from build123d import *

# Parameters (mm, degrees)
SKETCH1_W                      = 552
SKETCH1_H                      = 450
BOSS_EXTRUDE1_DEPTH            = 100
SKETCH2_W                      = 97
SKETCH2_H                      = 450
CUT_EXTRUDE1_DEPTH             = 90
SKETCH3_W                      = 450
SKETCH3_H                      = 97
CUT_EXTRUDE2_DEPTH             = 90
BOSS_EXTRUDE2_DEPTH            = 3
SKETCH5_W                      = 360
SKETCH5_H                      = 100
CUT_EXTRUDE3_DEPTH             = 542.403325206
SKETCH6_W                      = 20
SKETCH6_H                      = 3
BOSS_EXTRUDE3_DEPTH            = 90
SKETCH7_W                      = 20
SKETCH7_H                      = 3
BOSS_EXTRUDE4_DEPTH            = 90
CUT_EXTRUDE4_REACH             = 653.826
SKETCH9_W                      = 75
SKETCH9_H                      = 133
CUT_EXTRUDE5_DEPTH             = 538.285771261
CUT_EXTRUDE6_REACH             = 655.929
CUT_EXTRUDE7_REACH             = 653.826
CUT_EXTRUDE8_REACH             = 655.929
SKETCH13_W                     = 56
SKETCH13_H                     = 10
CUT_EXTRUDE9_DEPTH             = 1
SKETCH14_W                     = 56
SKETCH14_H                     = 10
CUT_EXTRUDE10_DEPTH            = 1
SKETCH15_W                     = 56
SKETCH15_H                     = 10
CUT_EXTRUDE11_DEPTH            = 1
SKETCH16_W                     = 56
SKETCH16_H                     = 10
CUT_EXTRUDE12_DEPTH            = 1
F_3_3_3_3_DIAMETER_HOLE1_D     = 3.3
F_3_3_3_3_DIAMETER_HOLE1_DEPTH = 2
F_17_0_17_DIAMETER_HOLE1_D     = 17
F_17_0_17_DIAMETER_HOLE1_DEPTH = 3
F_17_0_17_DIAMETER_HOLE2_D     = 17
F_17_0_17_DIAMETER_HOLE2_DEPTH = 103
FILLET1_R                      = 3


with BuildPart() as part:
    # Sketch1 → Boss-Extrude1 (new body)
    with BuildSketch(Plane(origin=(0, 120.173044165, 0), x_dir=(1, 0, 0), z_dir=(0, 1, 0))):
        with Locations((0, -225)):
            Rectangle(SKETCH1_W, SKETCH1_H)
    extrude(amount=-BOSS_EXTRUDE1_DEPTH)

    # Sketch2 → Cut-Extrude1 (cut)
    with BuildSketch(Plane(origin=(-273, 0, 0), x_dir=(0, -1, 0), z_dir=(-1, 0, 0))):
        with Locations((-68.673044165, 225)):
            Rectangle(SKETCH2_W, SKETCH2_H)
    extrude(amount=-CUT_EXTRUDE1_DEPTH, mode=Mode.SUBTRACT)

    # Sketch3 → Cut-Extrude2 (cut)
    with BuildSketch(Plane(origin=(273, 0, 0), x_dir=(0, 0, -1), z_dir=(1, 0, 0))):
        with Locations((-225, 68.673044165)):
            Rectangle(SKETCH3_W, SKETCH3_H)
    extrude(amount=-CUT_EXTRUDE2_DEPTH, mode=Mode.SUBTRACT)

    # Sketch4 → Boss-Extrude2 (add)
    with BuildSketch(Plane.XZ.offset(-20.173044165)):
        Polygon((-273, 360), (-273, 0), (-276, 0), (-276, 450), (-273, 450), (-273, 380), (-183, 380), (-183, 450), (183, 450), (183, 90), (273, 90), (273, 450), (276, 450), (276, 0), (273, 0), (273, 70), (183, 70), (183, 0), (-183, 0), (-183, 360), align=None)
    extrude(amount=BOSS_EXTRUDE2_DEPTH)

    # Sketch5 → Cut-Extrude3 (cut, through all)
    with BuildSketch(Plane(origin=(0, 0, 0), x_dir=(-1, 0, 0), z_dir=(0, 0, -1))):
        with Locations((0, 70.173044165)):
            Rectangle(SKETCH5_W, SKETCH5_H)
    extrude(amount=-CUT_EXTRUDE3_DEPTH, mode=Mode.SUBTRACT)

    # Sketch6 → Boss-Extrude3 (add)
    with BuildSketch(Plane(origin=(-273, 0, 0), x_dir=(0, 0, -1), z_dir=(1, 0, 0))):
        with Locations((-80, 18.673044165)):
            Rectangle(SKETCH6_W, SKETCH6_H)
    extrude(amount=BOSS_EXTRUDE3_DEPTH)

    # Sketch7 → Boss-Extrude4 (add)
    with BuildSketch(Plane.ZY.offset(-273)):
        with Locations((370, 18.673044165)):
            Rectangle(SKETCH7_W, SKETCH7_H)
    extrude(amount=BOSS_EXTRUDE4_DEPTH)

    # Sketch8 → Cut-Extrude4 (cut, up to next)
    with BuildSketch(Plane(origin=(-180, 0, 0), x_dir=(0, 0, -1), z_dir=(1, 0, 0)), mode=Mode.PRIVATE) as cut_extrude4_sk1:
        with BuildLine():
            Line((-440, 48.173044165), (-420, 48.173044165))
            ThreePointArc((-420, 48.173044165), (-413, 55.173044165), (-420, 62.173044165))
            Line((-420, 62.173044165), (-440, 62.173044165))
            ThreePointArc((-440, 62.173044165), (-447, 55.173044165), (-440, 48.173044165))
        make_face()
    cut_extrude4_tool1 = extrude(cut_extrude4_sk1.sketch, amount=-CUT_EXTRUDE4_REACH, mode=Mode.PRIVATE) & part.part
    add(cut_extrude4_tool1.solids().sort_by_distance((-180, 55.173044, 430))[0], mode=Mode.SUBTRACT)

    # Sketch9 → Cut-Extrude5 (cut, through all)
    with BuildSketch(Plane.XZ.offset(-117.173044165)):
        with Locations((-225, 225)):
            Rectangle(SKETCH9_W, SKETCH9_H)
    extrude(amount=-CUT_EXTRUDE5_DEPTH, mode=Mode.SUBTRACT)

    # Sketch10 → Cut-Extrude6 (cut, up to next)
    with BuildSketch(Plane.ZY.offset(183), mode=Mode.PRIVATE) as cut_extrude6_sk1:
        with BuildLine():
            Line((10, 48.173044165), (30, 48.173044165))
            ThreePointArc((30, 48.173044165), (37, 55.173044165), (30, 62.173044165))
            Line((30, 62.173044165), (10, 62.173044165))
            ThreePointArc((10, 62.173044165), (3, 55.173044165), (10, 48.173044165))
        make_face()
    cut_extrude6_tool1 = extrude(cut_extrude6_sk1.sketch, amount=-CUT_EXTRUDE6_REACH, mode=Mode.PRIVATE) & part.part
    add(cut_extrude6_tool1.solids().sort_by_distance((-183, 55.173044, 20))[0], mode=Mode.SUBTRACT)

    # Sketch11 → Cut-Extrude7 (cut, up to next)
    with BuildSketch(Plane.ZY.offset(-180), mode=Mode.PRIVATE) as cut_extrude7_sk1:
        with BuildLine():
            Line((440, 62.173044165), (420, 62.173044165))
            ThreePointArc((420, 62.173044165), (413, 55.173044165), (420, 48.173044165))
            Line((420, 48.173044165), (440, 48.173044165))
            ThreePointArc((440, 48.173044165), (447, 55.173044165), (440, 62.173044165))
        make_face()
    cut_extrude7_tool1 = extrude(cut_extrude7_sk1.sketch, amount=-CUT_EXTRUDE7_REACH, mode=Mode.PRIVATE) & part.part
    add(cut_extrude7_tool1.solids().sort_by_distance((180, 55.173044, 430))[0], mode=Mode.SUBTRACT)

    # Sketch12 → Cut-Extrude8 (cut, up to next)
    with BuildSketch(Plane(origin=(183, 0, 0), x_dir=(0, 0, -1), z_dir=(1, 0, 0)), mode=Mode.PRIVATE) as cut_extrude8_sk1:
        with BuildLine():
            Line((-10, 62.173044165), (-30, 62.173044165))
            ThreePointArc((-30, 62.173044165), (-37, 55.173044165), (-30, 48.173044165))
            Line((-30, 48.173044165), (-10, 48.173044165))
            ThreePointArc((-10, 48.173044165), (-3, 55.173044165), (-10, 62.173044165))
        make_face()
    cut_extrude8_tool1 = extrude(cut_extrude8_sk1.sketch, amount=-CUT_EXTRUDE8_REACH, mode=Mode.PRIVATE) & part.part
    add(cut_extrude8_tool1.solids().sort_by_distance((183, 55.173044, 20))[0], mode=Mode.SUBTRACT)

    # Sketch13 → Cut-Extrude9 (cut)
    with BuildSketch(Plane(origin=(0, 20.173044165, 0), x_dir=(-1, 0, 0), z_dir=(0, 1, 0))):
        with Locations((233, 80)):
            Rectangle(SKETCH13_W, SKETCH13_H)
    extrude(amount=-CUT_EXTRUDE9_DEPTH, mode=Mode.SUBTRACT)

    # Sketch14 → Cut-Extrude10 (cut)
    with BuildSketch(Plane(origin=(0, 20.173044165, 0), x_dir=(-1, 0, 0), z_dir=(0, 1, 0))):
        with Locations((233, 370)):
            Rectangle(SKETCH14_W, SKETCH14_H)
    extrude(amount=-CUT_EXTRUDE10_DEPTH, mode=Mode.SUBTRACT)

    # Sketch15 → Cut-Extrude11 (cut)
    with BuildSketch(Plane(origin=(0, 20.173044165, 0), x_dir=(-1, 0, 0), z_dir=(0, 1, 0))):
        with Locations((-233, 370)):
            Rectangle(SKETCH15_W, SKETCH15_H)
    extrude(amount=-CUT_EXTRUDE11_DEPTH, mode=Mode.SUBTRACT)

    # Sketch16 → Cut-Extrude12 (cut)
    with BuildSketch(Plane(origin=(0, 20.173044165, 0), x_dir=(-1, 0, 0), z_dir=(0, 1, 0))):
        with Locations((-233, 80)):
            Rectangle(SKETCH16_W, SKETCH16_H)
    extrude(amount=-CUT_EXTRUDE12_DEPTH, mode=Mode.SUBTRACT)

    # Ø3.3 (3.3) Diameter Hole1
    with Locations(Plane(origin=(0, 19.173044165, 0), x_dir=(1, 0, 0), z_dir=(0, 1, 0))):
        with Locations((-254.5, -80), (-211.5, -80), (-254.5, -370), (-211.5, -370), (211.5, -370), (254.5, -370), (211.5, -80), (254.5, -80)):
            Hole(F_3_3_3_3_DIAMETER_HOLE1_D / 2, depth=F_3_3_3_3_DIAMETER_HOLE1_DEPTH)

    # Ø17.0 (17) Diameter Hole1
    with Locations(Plane(origin=(0, 120.173044165, 0), x_dir=(1, 0, 0), z_dir=(0, 1, 0))):
        with Locations((225, -95)):
            Hole(F_17_0_17_DIAMETER_HOLE1_D / 2, depth=F_17_0_17_DIAMETER_HOLE1_DEPTH)

    # Ø17.0 (17) Diameter Hole2
    with Locations(Plane(origin=(0, 120.173044165, 0), x_dir=(1, 0, 0), z_dir=(0, 1, 0))):
        with Locations((-225, -100), (-225, -125), (-225, -325), (-225, -350)):
            Hole(F_17_0_17_DIAMETER_HOLE2_D / 2, depth=F_17_0_17_DIAMETER_HOLE2_DEPTH)

    # Fillet1
    fillet1_edges = [part.edges().sort_by_distance(p)[0] for p in [
        (-180, 120.173044165, 225),
        (180, 120.173044165, 225),
        (276, 120.173044165, 225),
        (-276, 120.173044165, 225),
    ]]
    fillet(fillet1_edges, radius=FILLET1_R)


solid = part.part
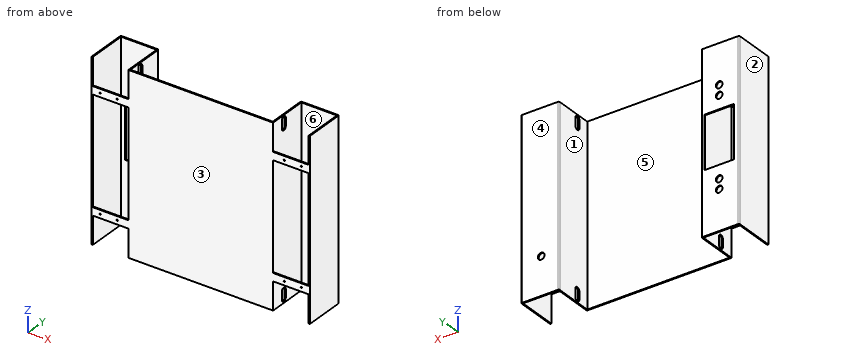
Design review of the part built by this model. Coordinates are the model's own, in mm. Face numbers are marked on the shaded views. A direction names the side the tool comes from. Round coordinates to 2 decimals unless told otherwise and drop trailing zeros. Loops run counter-clockwise (first coordinate to the right, second up) from the corner with the lowest first, then second, coordinate; pieces in that order, holes last. Notation, with made-up numbers: (-19.75, -3) - (12.25, -3) arc R13 cw to (12.25, 20) - close; hole circle Ø10 at (78, 69.5). An arc over 180 degrees is marked (long way). One line per item, written item: value. Start each with the question number.
1) Insertion check: pin 1 Ø22 at (x, z) = (-225, 325) entering from +Y; pin 2 Ø2.5 at (x, y) = (207.5, 19) entering from +Z; pin 3 Ø0.8 at (x, y) = (223.5, 19.5) entering from -Z; pin 4 Ø1.5 at (x, z) = (-172.5, 222.5) entering from +Y. Each pin has a flat end and moves straight along its axis. Give the tip position at first contact, or say it passes through.
2) Consider section C-C on x = 225. Give the boundary of the cut face in (y, z), then the cut area to 3 significant figures.
3) Consider section B-B on y = 41. Give the boundary of the cut face in (x, z).
4) Draft analysis for pull direction X (two halves, no side actions). For the marked faces 1, 2 and 3, state which applies: +X half, -X half, draft (parallel to the pull), parting line (faces both ways), or undercut.
5) Consider section D-D on x = -225. Give the number of separate pieces and of enclosed holes in the cut face, then the cut area to 3 significant figures.
6) For the marked faces 4, 5 and 6, list the 3-axis set-ups (+Z, -Z, +X, -X, +Y, -Y) from which the entire face can be reached by the end or side of a thin tool; tool diameter is ignored.
7) To check wall thickness, follow L1, parallel to X at y = 73.5, z = 118.5; L2, parallel to Z at x = -211.5, y = 18.7; L3, parallel to X at y = 18, z = 370. State the ranges of each line that lie inside material, in increasing order. Write a range as from..to.
8) Consider section A-A on z = 125. Give the boundary of the cut face in (x, y).
Reported:
1. pin 1: stops at y = 120.17
1. pin 2: stops at z = 380
1. pin 3: stops at z = 70
1. pin 4: stops at y = 20.17
2. outline: (17.17, 70) - (20.17, 70) - (20.17, 75) - (19.17, 75) - (19.17, 85) - (20.17, 85) - (20.17, 90) - (17.17, 90) - close; (17.17, 360) - (20.17, 360) - (20.17, 365) - (19.17, 365) - (19.17, 375) - (20.17, 375) - (20.17, 380) - (17.17, 380) - close; (117.17, 0) - (120.17, 0) - (120.17, 86.5) - (117.17, 86.5) - close; (117.17, 103.5) - (120.17, 103.5) - (120.17, 450) - (117.17, 450) - close
2. area: 1,400 mm^2
3. outline: (-276, 0) - (-273, 0) - (-273, 450) - (-276, 450) - close; (-183, 0) - (-180, 0) - (-180, 450) - (-183, 450) - close; (180, 0) - (183, 0) - (183, 450) - (180, 450) - close; (273, 0) - (276, 0) - (276, 450) - (273, 450) - close
4. face 1: undercut
4. face 2: -X half
4. face 3: draft
5. separate pieces: 8
5. enclosed holes: 0
5. area: 847 mm^2
6. face 4: +Z, -Z, +X, -X, +Y
6. face 5: +Z, -Z, +Y
6. face 6: +Z, -Z
7. L1: x = -276..-273, -183..-180, 180..183, 273..276
7. L2: z = 70..78.35, 81.65..90, 360..368.35, 371.65..380
7. L3: x = -276..-256.15, -252.85..-213.15, -209.85..209.85, 213.15..252.85, 256.15..276
8. outline: (-276, 17.17) - (-273, 17.17) - (-273, 117.17) - (-233.5, 117.17) - (-233.5, 120.17) - (-273, 120.17) arc R3 ccw to (-276, 117.17) - close; (-216.5, 117.17) - (-183, 117.17) - (-183, 17.17) - (183, 17.17) - (183, 117.17) - (273, 117.17) - (273, 17.17) - (276, 17.17) - (276, 117.17) arc R3 ccw to (273, 120.17) - (183, 120.17) arc R3 ccw to (180, 117.17) - (180, 20.17) - (-180, 20.17) - (-180, 117.17) arc R3 ccw to (-183, 120.17) - (-216.5, 120.17) - close
